from build123d import *

# Parameters (mm, degrees)
SKETCH4_W           = 93.22
SKETCH4_H           = 40.64
BOSS_EXTRUDE1_DEPTH = 10
SKETCH5_R           = 3.8
CUT_EXTRUDE1_DEPTH  = 3.9878
SKETCH6_R           = 2.05
CUT_EXTRUDE2_DEPTH  = 7.7978
SKETCH7_R           = 2.05
CUT_EXTRUDE5_DEPTH  = 7.7978


with BuildPart() as part:
    # Sketch4 → Boss-Extrude1 (new body)
    with BuildSketch(Plane.XY):
        Polygon((186.44, -13.916292355), (181.36, -21.916292355), (139.83, -21.916292355), (98.3, -21.916292355), (93.22, -13.916292355), align=None)
        with Locations((139.83, 6.403707645)):
            Rectangle(SKETCH4_W, SKETCH4_H)
    extrude(amount=BOSS_EXTRUDE1_DEPTH)

    # Sketch5 → Cut-Extrude1 (cut)
    with BuildSketch(Plane.XY.offset(10)):
        with Locations((118.62, 6.403707645)):
            Circle(SKETCH5_R)
        with Locations((161.04, 6.403707645)):
            Circle(SKETCH5_R)
    extrude(amount=-CUT_EXTRUDE1_DEPTH, mode=Mode.SUBTRACT)

    # Sketch6 → Cut-Extrude2 (cut)
    with BuildSketch(Plane.XY.offset(6.0122)):
        with Locations((118.62, 6.403707645)):
            Circle(SKETCH6_R)
    extrude(amount=-CUT_EXTRUDE2_DEPTH, mode=Mode.SUBTRACT)

    # Sketch7 → Cut-Extrude5 (cut)
    with BuildSketch(Plane.XY.offset(6.0122)):
        with Locations((161.04, 6.403707645)):
            Circle(SKETCH7_R)
    extrude(amount=-CUT_EXTRUDE5_DEPTH, mode=Mode.SUBTRACT)


solid = part.part
Here's how the part is built. I have some questions about the finished solid (model axes, mm). A direction names the side the tool comes from. Give positions to 0.01 mm unless a question says otherwise; leave off trailing zeros. Order: outer loops, then holes, each group sorted by start corner. A loop starts at its lowest first (then second) coordinate and runs counter-clockwise, first axis right, second up. Notation, with made-up numbers: (44.25, 8.25) -> (86.25, 8.25) arc R22 ccw to (86.25, 30.25) -> close; hole circle Ø11 at (46, 55). An arc over 180 degrees is marked (long way). One line per item, written item: value. Start each with the question number.
1. I need wall thicknesses on probe 1 along Y at (x, z) = (161.04, 8.3); probe 2 along X at (y, z) = (7, 1); probe 3 along Y at (x, z) = (161, 5.75). Which ranges of each line are inside material? Lowest first, please. Write a range as from..to.
2. We'd pull the mould along X, two halves only. Please class faces 1 (the face through (164.55, 4.95, 8.03)), 2 (the face through (140, 3, 0)), 3 (the face through (186.44, 6, 5)), 4 (the face through (95.796, -17.972, 4.93)): released by +X, released by -X, zero draft, split by the parting line, or undercut.
3. Imagine slicing it at A-A, the plane x = 118.62. List the corners of the cut face in (y, z) for me.
4. Imagine slicing it at B-B, the plane z = 7.5. List the corners of the cut face in (x, y) for me, plus the area to 3 significant figures.
5. Will these pins go through, and if not, where does the flat tip stop? pin 1 Ø3.5 at (x, y) = (118.62, 6.4) entering from -Z; pin 2 Ø4 at (x, y) = (160, 6) entering from +Z.
6. For faces 5 (the face through (139, 26.724, 5)), 6 (the face through (163, 5, 6.012)), which set-ups out of +Z, -Z, +X, -X, +Y, -Y let a thin tool reach every point of the face, with its end or its side?
Values follow:
1. probe 1: y = -21.92..2.6, 10.2..26.72
1. probe 2: x = 93.22..116.66, 120.58..159.08, 163..186.44
1. probe 3: y = -21.92..4.35, 8.45..26.72
2. face 1: undercut
2. face 2: zero draft
2. face 3: released by +X
2. face 4: released by -X
3. outline: (-21.92, 0) -> (4.35, 0) -> (4.35, 6.01) -> (2.6, 6.01) -> (2.6, 10) -> (-21.92, 10) -> close; (8.45, 0) -> (26.72, 0) -> (26.72, 10) -> (10.2, 10) -> (10.2, 6.01) -> (8.45, 6.01) -> close
4. outline: (93.22, -13.92) -> (98.3, -21.92) -> (181.36, -21.92) -> (186.44, -13.92) -> (186.44, 26.72) -> (93.22, 26.72) -> close; hole circle Ø7.6 at (118.62, 6.4); hole circle Ø7.6 at (161.04, 6.4)
4. area: 4,400 mm2
5. pin 1: passes through
5. pin 2: stops at z = 6.01
6. face 5: +Z, -Z, +X, -X, +Y
6. face 6: +Z
